Input: part model. Units: mm. Frame: model coordinates. Face numbers are marked on the shaded views. A direction names the side the tool comes from. Give positions to 0.01 mm unless a question says otherwise; leave off trailing zeros. Write each loop counter-clockwise with the first axis right and the second up, starting at its lowest first coordinate (ties: lowest second). Pieces come first, ordered by that corner, then holes. Notation, with made-up numbers: (21.25, 14) - (71.25, 14) arc R32 ccw to (71.25, 52) - close; hole circle Ø6 at (10, 59.5). An arc over 180 degrees is marked (long way). Use a Markdown table: item, result. Add a question column.
1. Section query A-A, the plane y = 0. Return loops of the section in (x, z), plus the area to 3 significant figures.
2. Section query C-C, the plane x = -1.5. Return loops of the section in (y, z), plus the area to 3 significant figures.
3. Material intervals for probe 1 along Z at (x, y) = (4.5, 0); probe 2 along Y at (x, z) = (-1.75, 17.5); probe 3 along Z at (x, y) = (1.75, 3.5), sorted ascending.
4. Section query B-B, the plane z = 172.5. Return loops of the section in (x, y), plus the area to 3 significant figures.
5. Set-up query: the marked faces 1, 2 and 3. Return all of +Z, -Z, +X, -X, +Y, -Y with unobstructed straight access to the full face (end or side cutting, diameter ignored); none if empty.
6. Section query D-D, the plane y = 13.5. Return loops of the section in (x, z).
7. Pin query (flat end, axial travel): pin 1 (11.5 mm diameter, centred on y = 0, z = 17.5, fed in from -X); pin 2 (0.8 mm diameter, centred on x = -4.5, y = -6.5, fed in from -Z); pin 3 (0.8 mm diameter, centred on x = -4.5, y = -2, fed in from +Z). Return the tip coordinate at first contact, or that it passes through.
Autodesk Inventor part; units mm, degrees
ref_plane "Startebene" through (0, 0, 0) normal (0, 0, 1) x (1, 0, 0)
ref_plane "Endebene" through (0, 0, 190) normal (0, 0, 1) x (1, 0, 0)
ref_plane "YZ Plane" through (0, 0, 0) normal (1, 0, 0) x (0, 1, 0)
ref_plane "Startebene" through (0, 0, 0) normal (0, 0, 1) x (1, 0, 0)
ref_plane "Endebene" through (0, 0, 190) normal (0, 0, 1) x (1, 0, 0)
sketch "Skizze" plane through (0, 0, 0) normal (0, 0, 1) x (1, 0, 0)
  line L0 (5, -17.5) -> (-5, -17.5)
  line L1 (-5, -17.5) -> (-5, 17.5)
  line L2 (-5, 17.5) -> (5, 17.5)
  line L3 (5, 17.5) -> (5, -17.5)
  line L4 (-6, 0) -> (8, 0) construction
  line L5 (0, -30) -> (0, 40) construction
  line L6 (0, 54) -> (0, -44) construction
  line L7 (-9.2, 0) -> (13.2, 0) construction
  dimension "d0" = 35
  dimension "d1" = 10
  dimension "d4" = 5
  dimension "d5" = 17.5
extrude "Körper" add sketch "Skizze" along normal up to surface (190 mm away) from surface at 0
sketch "Sketch3" plane through (0, 0, 0) normal (0, 0, 1) x (1, 0, 0)
  line L0 (0, 0) -> (10, 0)
ref_plane "Work Plane3" through (0, 0, 0) normal (0, -1, 0) x (1, 0, 0)
sketch "Sketch4" plane through (0, 0, 0) normal (0, -1, 0) x (1, 0, 0)
  line L0 (-2, 0) -> (12, 0)
  line L1 (-2, 190) -> (12, 190)
  dimension "d9" = 190
sketch "Skizze5" plane through (5, -17.5, 190) normal (1, 0, 0) x (0, 0, -1)
  line L0 (0, 35) -> (0, 0)
  line L1 (190, 35) -> (190, 0)
  line L2 (190, 35) -> (0, 35)
  point P0 (190, 17.5)
  point P1 (17.5, 17.5)
  point P2 (172.5, 17.5)
  dimension "d10" = 17.5
  dimension "d11" = 17.5
  dimension "d12" = 17.5
  dimension "d13" = 17.5
hole "Bohrung1" at (5, 0, 17.5) at (5, 0, 172.5) direction (-1, 0, 0) diameter 10 end through all
sketch "Skizze7" plane through (-5, -17.5, 0) normal (0, -1, 0) x (1, 0, 0)
  line L0 (0, 190) -> (1, 190)
  line L1 (1, 190) -> (1, 155)
  line L2 (1, 155) -> (0, 155)
  line L3 (0, 155) -> (0, 190)
  line L4 (0, 0) -> (1, 0)
  line L5 (1, 0) -> (1, 35)
  line L6 (1, 35) -> (0, 35)
  line L7 (0, 35) -> (0, 0)
  dimension "d26" = 35
  dimension "d27" = 35
  dimension "d28" = 1
  dimension "d29" = 1
extrude "Extrusion2" cut sketch "Skizze7" against normal through all
equation "\"d0\" = G_W"
equation "\"d1\" = G_H"
equation "\"d4\" = 0.5 * d1"
equation "\"d5\" = 0.5 * d0"
equation "\"d2\" = G_L"
equation "\"G_W\" = 35"
equation "\"G_H\" = 10"
equation "\"G_L\" = d9"
equation "\"G_OFFSET_START\" = 0"
equation "\"G_OFFSET_END\" = 0"
properties part number "EN 10058 - 35 x 10 - 190" material "Stahl, weich"
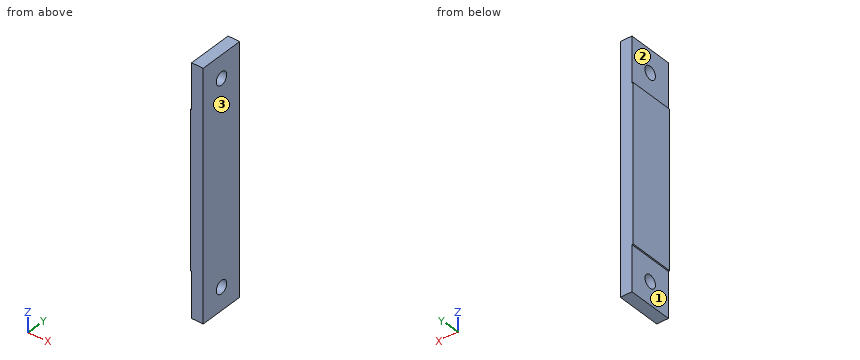
Result sheet:
| question | item | result |
|---|---|---|
| 1 | outline | (-5, 35) - (-4, 35) - (-4, 22.5) - (5, 22.5) - (5, 167.5) - (-4, 167.5) - (-4, 155) - (-5, 155) - close; (-4, 0) - (5, 0) - (5, 12.5) - (-4, 12.5) - close; (-4, 177.5) - (5, 177.5) - (5, 190) - (-4, 190) - close |
| 1 | area | 1,650 mm² |
| 2 | outline | (-17.5, 0) - (17.5, 0) - (17.5, 190) - (-17.5, 190) - close; hole circle Ø10 at (0, 17.5); hole circle Ø10 at (0, 172.5) |
| 2 | area | 6,490 mm² |
| 3 | probe 1 | z = 0 to 12.5, 22.5 to 167.5, 177.5 to 190 |
| 3 | probe 2 | y = -17.5 to -5, 5 to 17.5 |
| 3 | probe 3 | z = 0 to 13.93, 21.07 to 168.93, 176.07 to 190 |
| 4 | outline | (-4, -17.5) - (5, -17.5) - (5, -5) - (-4, -5) - close; (-4, 5) - (5, 5) - (5, 17.5) - (-4, 17.5) - close |
| 4 | area | 225 mm² |
| 5 | face 1 | -Z, -X, +Y, -Y |
| 5 | face 2 | +Z, -X, +Y, -Y |
| 5 | face 3 | +Z, -Z, +X, +Y, -Y |
| 6 | outline | (-5, 35) - (-4, 35) - (-4, 0) - (5, 0) - (5, 190) - (-4, 190) - (-4, 155) - (-5, 155) - close |
| 7 | pin 1 | stops at x = -4 |
| 7 | pin 2 | stops at z = 35 |
| 7 | pin 3 | stops at z = 155 |
